```python
from build123d import *

# Parameters (mm, degrees)
CYLINDER025_R          = 1.75
CYLINDER025_DEPTH      = 44
CYLINDER025_ROLL_ANGLE = 90
CYLINDER034_R          = 1.75
CYLINDER034_DEPTH      = 44
CYLINDER034_ROLL_ANGLE = 90
CYLINDER035_R          = 1.75
CYLINDER035_DEPTH      = 44
CYLINDER035_ROLL_ANGLE = 90
CYLINDER036_R          = 10
CYLINDER036_DEPTH      = 34
CYLINDER036_ROLL_ANGLE = 90
CYLINDER024_R          = 1.75
CYLINDER024_DEPTH      = 44
CYLINDER024_ROLL_ANGLE = 90
BOX052_W               = 7
BOX052_H               = 7.9
BOX052_DEPTH           = 17
BOX050_W               = 47
BOX050_H               = 6.1
BOX050_DEPTH           = 17
BOX051_W               = 7
BOX051_H               = 7.9
BOX051_DEPTH           = 17


with BuildPart() as cylinder_for_hole_10_groovemount_r001:
    # Cylinder025 → Cylinder025 (new body)
    with BuildSketch(Plane.XY):
        Circle(CYLINDER025_R)
    extrude(amount=CYLINDER025_DEPTH)


with BuildPart() as cylinder_for_hole_10_groovemount_r001_1:
    # Cylinder025 roll: moved
    add(cylinder_for_hole_10_groovemount_r001.part.rotate(Axis((0, 0, 0), (1, 0, 0)), CYLINDER025_ROLL_ANGLE))


with BuildPart() as cylinder_for_hole_10_groovemount_r001_2:
    # Cylinder025 placement: moved
    add(cylinder_for_hole_10_groovemount_r001_1.part.moved(Location((20, 6, -2.5))))


with BuildPart() as cylinder_for_hole_3_motherboard002:
    # Cylinder034 → Cylinder034 (new body)
    with BuildSketch(Plane.XY):
        Circle(CYLINDER034_R)
    extrude(amount=CYLINDER034_DEPTH)


with BuildPart() as cylinder_for_hole_3_motherboard002_1:
    # Cylinder034 roll: moved
    add(cylinder_for_hole_3_motherboard002.part.rotate(Axis((0, 0, 0), (1, 0, 0)), CYLINDER034_ROLL_ANGLE))


with BuildPart() as cylinder_for_hole_3_motherboard002_2:
    # Cylinder034 placement: moved
    add(cylinder_for_hole_3_motherboard002_1.part.moved(Location((-20, 6, -13.5))))


with BuildPart() as cylinder_for_hole_4_motherboard002:
    # Cylinder035 → Cylinder035 (new body)
    with BuildSketch(Plane.XY):
        Circle(CYLINDER035_R)
    extrude(amount=CYLINDER035_DEPTH)


with BuildPart() as cylinder_for_hole_4_motherboard002_1:
    # Cylinder035 roll: moved
    add(cylinder_for_hole_4_motherboard002.part.rotate(Axis((0, 0, 0), (1, 0, 0)), CYLINDER035_ROLL_ANGLE))


with BuildPart() as cylinder_for_hole_4_motherboard002_2:
    # Cylinder035 placement: moved
    add(cylinder_for_hole_4_motherboard002_1.part.moved(Location((20, 6, -13.5))))


with BuildPart() as obj1_hole:
    # Cylinder036 → Cylinder036 (new body)
    with BuildSketch(Plane.XY):
        Circle(CYLINDER036_R)
    extrude(amount=CYLINDER036_DEPTH)


with BuildPart() as obj1_hole_1:
    # Cylinder036 roll: moved
    add(obj1_hole.part.rotate(Axis((0, 0, 0), (1, 0, 0)), CYLINDER036_ROLL_ANGLE))


with BuildPart() as obj1_hole_2:
    # Cylinder036 placement: moved
    add(obj1_hole_1.part.moved(Location((4.5, 0, -4))))


with BuildPart() as obj2:
    # Cylinder024 → Cylinder024 (new body)
    with BuildSketch(Plane.XY):
        Circle(CYLINDER024_R)
    extrude(amount=CYLINDER024_DEPTH)


with BuildPart() as obj2_1:
    # Cylinder024 roll: moved
    add(obj2.part.rotate(Axis((0, 0, 0), (1, 0, 0)), CYLINDER024_ROLL_ANGLE))


with BuildPart() as obj2_2:
    # Cylinder024 placement: moved
    add(obj2_1.part.moved(Location((-20, 6, -2.5))))

    # Fusion009: union cylinder for hole 10 - Groovemount R001, cylinder for hole 3 - Motherboard002, cylinder for hole 4 - Motherboard002, obj1_hole
    add(cylinder_for_hole_10_groovemount_r001_2.part)
    add(cylinder_for_hole_3_motherboard002_2.part)
    add(cylinder_for_hole_4_motherboard002_2.part)
    add(obj1_hole_2.part)


with BuildPart() as obj3:
    # Box052 → Box052 (new body)
    with BuildSketch(Plane(origin=(-23.5, -12.9, -9), x_dir=(1, 0, 0), z_dir=(0, 0, 1))):
        with Locations((3.5, 3.95)):
            Rectangle(BOX052_W, BOX052_H)
    extrude(amount=BOX052_DEPTH)


with BuildPart() as obj1:
    # Box050 → Box050 (new body)
    with BuildSketch(Plane(origin=(-23.5, -19, -9), x_dir=(1, 0, 0), z_dir=(0, 0, 1))):
        with Locations((23.5, 3.05)):
            Rectangle(BOX050_W, BOX050_H)
    extrude(amount=BOX050_DEPTH)


with BuildPart() as obj4:
    # Box051 → Box051 (new body)
    with BuildSketch(Plane(origin=(16.5, -12.9, -9), x_dir=(1, 0, 0), z_dir=(0, 0, 1))):
        with Locations((3.5, 3.95)):
            Rectangle(BOX051_W, BOX051_H)
    extrude(amount=BOX051_DEPTH)

    # Fusion010: union obj3, obj1
    add(obj3.part)
    add(obj1.part)

    # Cut008: cut obj2
    add(obj2_2.part, mode=Mode.SUBTRACT)


solid = obj4.part
```
The model under review builds one solid part; all positions refer to its coordinate system, in mm. A direction names the side the tool comes from. Coordinates: 2 decimals unless noted, no trailing zeros. Loops run counter-clockwise (first coordinate to the right, second up) from the corner with the lowest first, then second, coordinate; pieces in that order, holes last. Notation, with made-up numbers: (61.25, 40) -> (87.25, 40) arc R34 cw to (87.25, 71) -> close; hole circle Ø2 at (26, -5.75). An arc over 180 degrees is marked (long way). Answer as CSV lines item,"result".
Item 1: Take a section at A-A, the plane y = -9. State the section outline as (x, z) points.
Results below:
outline,"(-23.5, -9) -> (-16.5, -9) -> (-16.5, 8) -> (-23.5, 8) -> close; (16.5, -9) -> (23.5, -9) -> (23.5, 8) -> (16.5, 8) -> close; hole circle Ø3.5 at (-20, -2.5); hole circle Ø3.5 at (20, -2.5)"
Item 2: Take a section at B-B, the plane x = -20. State the section outline as (y, z) points.
Results below:
outline,"(-19, -9) -> (-5, -9) -> (-5, -4.25) -> (-19, -4.25) -> close; (-19, -0.75) -> (-5, -0.75) -> (-5, 8) -> (-19, 8) -> close"
Item 3: Take a section at D-D, the plane y = -14.5. State the section outline as (x, z) points, and give its area (3 significant figures).
Results below:
outline,"(-23.5, -9) -> (-4.16, -9) arc R10 cw (long way) to (13.16, -9) -> (23.5, -9) -> (23.5, 8) -> (-23.5, 8) -> close; hole circle Ø3.5 at (-20, -2.5); hole circle Ø3.5 at (20, -2.5)"
area,"527 mm2"
Item 4: Take a section at C-C, the plane z = 5.5. State the section outline as (x, y) points.
Results below:
outline,"(-23.5, -19) -> (1.38, -19) -> (1.38, -12.9) -> (-16.5, -12.9) -> (-16.5, -5) -> (-23.5, -5) -> close; (7.62, -19) -> (23.5, -19) -> (23.5, -5) -> (16.5, -5) -> (16.5, -12.9) -> (7.62, -12.9) -> close"
Item 5: Draft analysis for pull direction X (two halves, no side actions). For faces 1 (the flat face through (23.5, -12, -1)), 2 (the flat face through (-6, -19, -1)), 3 (the flat face through (16.5, -9, -1)), state which applies: +X half, -X half, draft (parallel to the pull), parting line (faces both ways), or undercut.
Results below:
face 1,"+X half"
face 2,"draft"
face 3,"undercut"
Item 6: Machinability: for faces 4 (the flat face through (-20.8, -5, -0.6)), 5 (the flat face through (-16.5, -9, -1)), which of the approach directions +Z, -Z, +X, -X, +Y, -Y give a long, thin tool a straight path to every point of the face, cutting with its end or side? Answer none if there is none.
Results below:
face 4,"+Z, -Z, +X, -X, +Y"
face 5,"+Z, -Z, +Y"
Item 7: Insertion check: pin 1 (8.5 mm diameter, centred on x = -5, z = -3.5, fed in from +Y). The pin has a flat end and moves straight along its axis. Give the tip position at first contact, or say it passes through.
Results below:
pin 1,"stops at y = -12.9"
Item 8: For L1, parallel to X at y = -11.5, z = -1.5; L2, parallel to X at y = -12.25, z = 5.75; L3, parallel to X at y = -12, z = -2, list the stretches that pass through material, from the lowest coordinate up.
Results below:
L1,"x = -23.5 to -21.44, -18.56 to -16.5, 16.5 to 18.56, 21.44 to 23.5"
L2,"x = -23.5 to -16.5, 16.5 to 23.5"
L3,"x = -23.5 to -21.68, -18.32 to -16.5, 16.5 to 18.32, 21.68 to 23.5"
